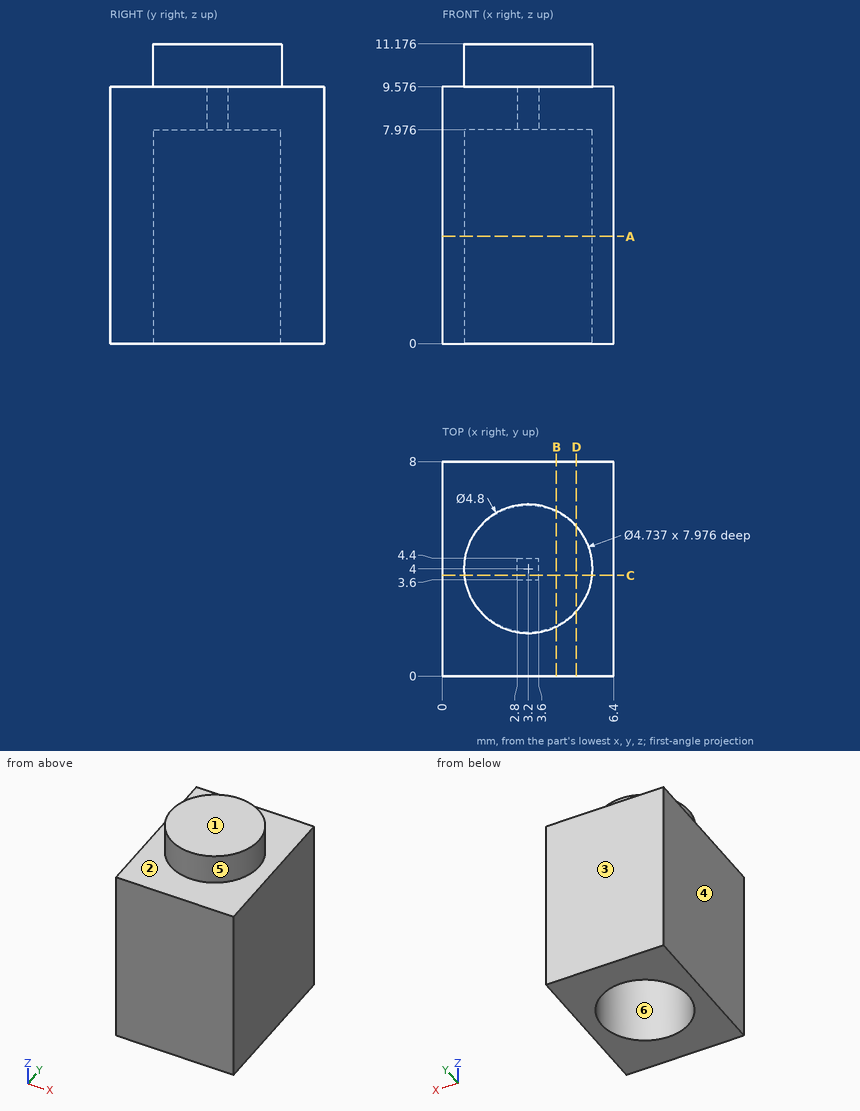
Can you work these out from the drawing? Everything is in mm from the part's minimum corner. A direction names the side the tool comes from. Round coordinates to 2 decimals unless told otherwise and drop trailing zeros. Loops run counter-clockwise (first coordinate to the right, second up) from the corner with the lowest first, then second, coordinate; pieces in that order, holes last. Notation, with made-up numbers: (29, 17.5) - (67, 17.5) arc R33 ccw to (67, 50.5) - close; hole circle Ø1 at (52.25, 73.25). An arc over 180 degrees is marked (long way). One line per question, with ' | ' between items. Start each with the question number.
Q1. I want a section at A-A (z = 4). Write out the boundary of the cut face in (x, y).
Q2. I want a section at C-C (y = 3.75). Write out the boundary of the cut face in (x, z) (1 decimal).
Q3. I want a section at D-D (x = 5). Write out the boundary of the cut face in (y, z).
Q4. We'd pull the mould along Y, two halves only. Please class the marked faces 3, 4, 5 and 6: +Y half, -Y half, draft (parallel to the pull), parting line (faces both ways), or undercut.
Q5. For the marked faces 1 and 2, which set-ups out of +Z, -Z, +X, -X, +Y, -Y let a thin tool reach every point of the face, with its end or its side?
Q6. Please list where these lines run through material, in increasing order: line 1 (Z direction, x = 4.5, y = 1.25); line 2 (Z direction, x = 3.25, y = 2); line 3 (Y direction, x = 5.25, z = 6) (1 decimal). Write a range as [from, to].
Q7. I want a section at B-B (x = 4.25). Write out the boundary of the cut face in (y, z).
Response values:
1) outline: (0, 0) - (6.4, 0) - (6.4, 8) - (0, 8) - close; hole circle Ø4.74 at (3.2, 4)
2) outline: (0, 0) - (0.8, 0) - (0.8, 8) - (2.8, 8) - (2.8, 9.6) - (3.6, 9.6) - (3.6, 8) - (5.6, 8) - (5.6, 0) - (6.4, 0) - (6.4, 9.6) - (5.6, 9.6) - (5.6, 11.2) - (0.8, 11.2) - (0.8, 9.6) - (0, 9.6) - close
3) outline: (0, 0) - (2.46, 0) - (2.46, 7.98) - (5.54, 7.98) - (5.54, 0) - (8, 0) - (8, 9.58) - (5.59, 9.58) - (5.59, 11.18) - (2.41, 11.18) - (2.41, 9.58) - (0, 9.58) - close
4) face 3: +Y half | face 4: draft | face 5: parting line | face 6: undercut
5) face 1: +Z, +X, -X, +Y, -Y | face 2: +Z
6) line 1: z = [0, 9.58] | line 2: z = [7.98, 11.18] | line 3: y = [0, 2.8], [5.2, 8]
7) outline: (0, 0) - (1.88, 0) - (1.88, 7.98) - (6.12, 7.98) - (6.12, 0) - (8, 0) - (8, 9.58) - (6.16, 9.58) - (6.16, 11.18) - (1.84, 11.18) - (1.84, 9.58) - (0, 9.58) - close
